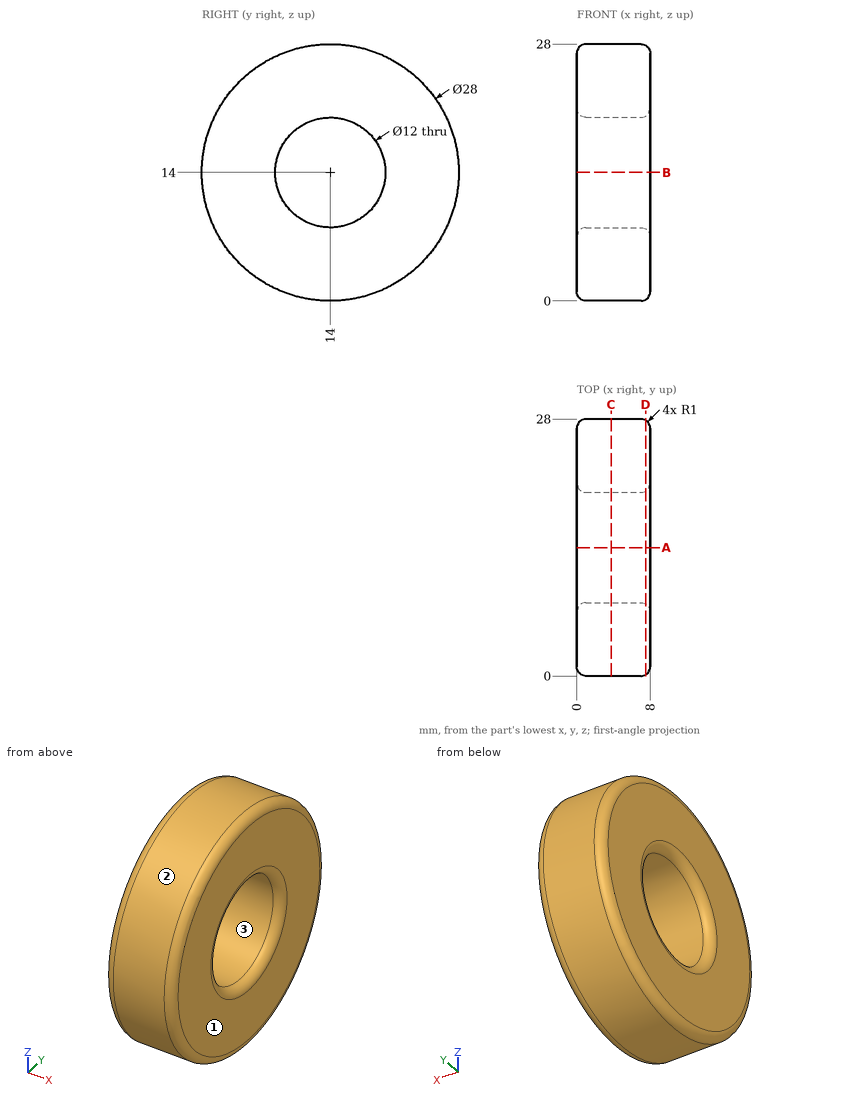
Check sheet for the drawn part. Datum: minimum x, y, z corner. Units: mm. Round coordinates to 2 decimals unless told otherwise and drop trailing zeros. Write each loop counter-clockwise with the first axis right and the second up, starting at its lowest first coordinate (ties: lowest second). Pieces come first, ordered by that corner, then holes. Notation, with made-up numbers: (59.5, 55) -> (83.5, 55) arc R29 ccw to (83.5, 84) -> close; hole circle Ø9 at (22, 41). An arc over 180 degrees is marked (long way). One line per item, written item: value. Start each with the question number.
(1) Cross-section at D-D, the plane x = 7.5. Record the cut outline in (y, z), and give its area (3 significant figures).
(2) Go/stop test with flat-tipped pins: pin 1 Ø4 at (x, z) = (2, 24) entering from -Y; pin 2 Ø3 at (x, y) = (3, 11) entering from +Z; pin 3 Ø3 at (x, y) = (2.5, 22.5) entering from +Z. Record where each tip stops, or that it passes through.
(3) Draft check along Y on the marked faces 1, 2 and 3. Enter one of: +Y half, -Y half, draft (parallel to the pull), parting line (faces both ways), or undercut.
(4) Cross-section at C-C, the plane x = 3.75. Record the cut outline in (y, z).
(5) Scan lines: line 1 (Z direction, x = 4.3, y = 14); line 2 (Z direction, x = 2.75, y = 10.5). Record each from-to range of solid material in increasing order. Write a range as [from, to].
(6) Cross-section at A-A, the plane y = 14. Record the cut outline in (x, z).
Answer:
1. outline: circle Ø27.73 at (14, 14); hole circle Ø12.27 at (14, 14)
1. area: 486 mm²
2. pin 1: y = 2.51
2. pin 2: z = 27.92
2. pin 3: z = 26.12
3. face 1: draft
3. face 2: parting line
3. face 3: undercut
4. outline: circle Ø28 at (14, 14); hole circle Ø12 at (14, 14)
5. line 1: [0, 8], [20, 28]
5. line 2: [0.44, 9.13], [18.87, 27.56]
6. outline: (0, 1) arc R1 ccw to (1, 0) -> (7, 0) arc R1 ccw to (8, 1) -> (8, 7) arc R1 ccw to (7, 8) -> (1, 8) arc R1 ccw to (0, 7) -> close; (0, 21) arc R1 ccw to (1, 20) -> (7, 20) arc R1 ccw to (8, 21) -> (8, 27) arc R1 ccw to (7, 28) -> (1, 28) arc R1 ccw to (0, 27) -> close
